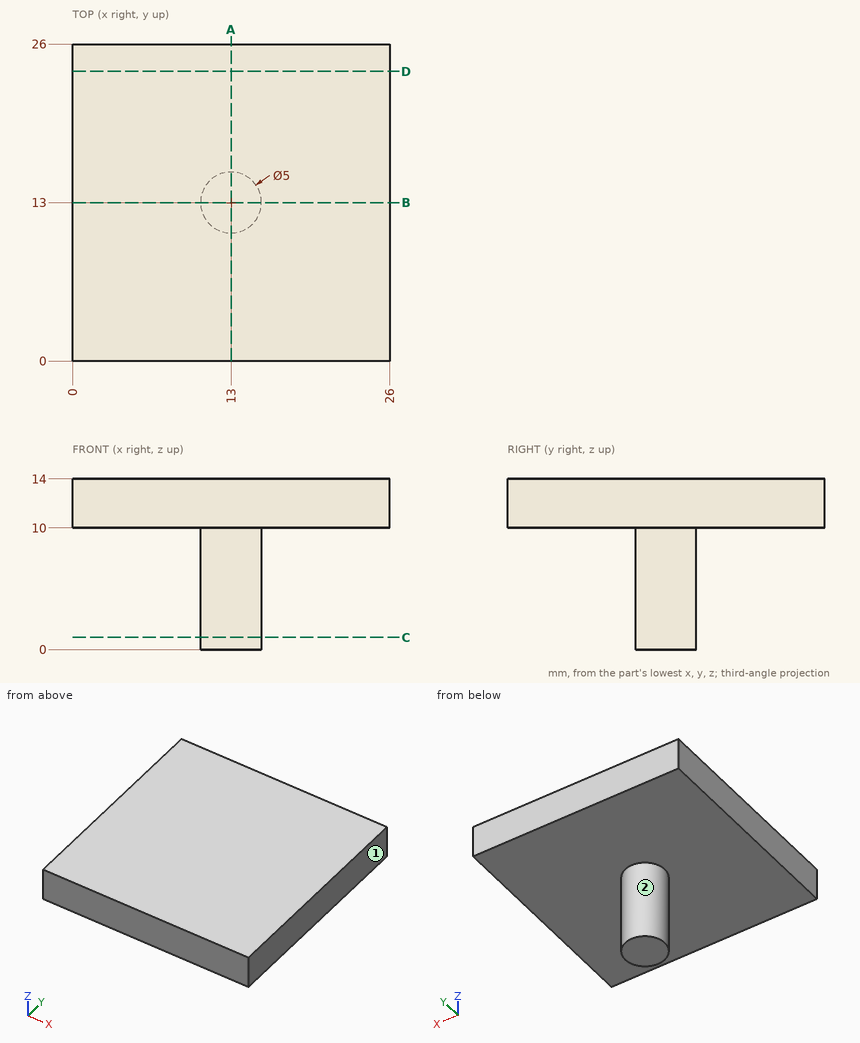
Input: dimensioned drawing with shaded views. Units: mm. Origin: part minimum x, y, z. A direction names the side the tool comes from. Coordinates: 2 decimals unless noted, no trailing zeros. Write each loop counter-clockwise with the first axis right and the second up, starting at its lowest first coordinate (ties: lowest second). Pieces come first, ordered by that corner, then holes. Notation, with made-up numbers: M 27,53.5 L 78,53.5 A18 cw 78,73.5 Z; hole C 69.25,-29.5 d7. An arc over 180 degrees is marked long. Answer as a JSON object with one key per item and string values. Group by question number.
(1) Section A-A on x = 13. Output: boundary loops of the cut face in (y, z), plus the area to 3 significant figures.
(2) Ray query, line 1 along Z through (x, y) = (13, 9); line 2 along Y through (x, z) = (14, 6.25); line 3 along X through (y, z) = (12.25, 4.25). Return the intervals inside material, ascending. Write a range as [from, to].
(3) Contact query for flat-ended pins moving along their axis: P1, Ø1, axis at y = 13, z = 3, coming from the +X side; P2, Ø3, axis at x = 12, y = 15, coming from the -Z side; P3, Ø12, axis at x = 9, y = 3, coming from the -Z side. Output: stop coordinate, or through.
(4) Set-up query: the marked faces 1 and 2. Return all of +Z, -Z, +X, -X, +Y, -Y with unobstructed straight access to the full face (end or side cutting, diameter ignored); none if empty.
(5) Section D-D on y = 23.75. Output: boundary loops of the cut face in (x, z), plus the area to 3 significant figures.
(6) Section C-C on z = 1. Output: boundary loops of the cut face in (x, y).
Result set:
{
 "1": {"outline": "M 0,10 L 10.5,10 L 10.5,0 L 15.5,0 L 15.5,10 L 26,10 L 26,14 L 0,14 Z", "area": "154 mm2"},
 "2": {"line 1": "z = [10, 14]", "line 2": "y = [10.71, 15.29]", "line 3": "x = [10.62, 15.38]"},
 "3": {"P1": "stops at x = 15.5", "P2": "stops at z = 0", "P3": "stops at z = 10"},
 "4": {"face 1": "+Z, -Z, +X, +Y, -Y", "face 2": "-Z"},
 "5": {"outline": "M 0,10 L 26,10 L 26,14 L 0,14 Z", "area": "104 mm2"},
 "6": {"outline": "C 13,13 d5"}
}
